Check sheet for the modelled part. Datum: model origin and axes. Units: mm. A direction names the side the tool comes from. Give positions to 0.01 mm unless a question says otherwise; leave off trailing zeros. Order: outer loops, then holes, each group sorted by start corner. A loop starts at its lowest first (then second) coordinate and runs counter-clockwise, first axis right, second up.
from build123d import *

# Parameters (mm, degrees)
F1_DEPTH  = 114.3
F2_DEPTH  = 12.7
F4_DEPTH  = 6.35
F5_W      = 6.35
F5_H      = 6.35
F6_DEPTH  = 6.35
F7_W      = 6.35
F7_H      = 6.35
F8_DEPTH  = 6.35
F9_R      = 2.5
F10_DEPTH = 6.35
F11_R     = 2.5
F12_DEPTH = 6.35
F13_W     = 6.35
F13_H     = 6.35
F14_DEPTH = 6.35


with BuildPart() as f1:
    # F0 (on Front) → F1 (new body)
    with BuildSketch(Plane.XZ):
        Polygon((45.4323484187, 0), (22.7161742094, 39.3455678842), (-22.7161742094, 39.3455678842), (-45.4323484187, 0), (-22.7161742094, -39.3455678842), (22.7161742094, -39.3455678842), align=None)
        Polygon((38.1, 0), (19.05, -32.9955678842), (-19.05, -32.9955678842), (-38.1, 0), (-19.05, 32.9955678842), (19.05, 32.9955678842), align=None, mode=Mode.SUBTRACT)
    extrude(amount=F1_DEPTH)

    # F0 (on Front) → F2 (join)
    with BuildSketch(Plane.XZ):
        Polygon((45.4323484187, 0), (22.7161742094, 39.3455678842), (-22.7161742094, 39.3455678842), (-45.4323484187, 0), (-22.7161742094, -39.3455678842), (22.7161742094, -39.3455678842), align=None)
        Polygon((38.1, 0), (19.05, -32.9955678842), (-19.05, -32.9955678842), (-38.1, 0), (-19.05, 32.9955678842), (19.05, 32.9955678842), align=None, mode=Mode.SUBTRACT)
    extrude(amount=-F2_DEPTH)

    # F3 (on Front) → F4 (join)
    with BuildSketch(Plane.XZ):
        Polygon((19.05, -32.9955678842), (38.1, 0), (19.05, 32.9955678842), (-19.05, 32.9955678842), (-38.1, 0), (-19.05, -32.9955678842), align=None)
    extrude(amount=F4_DEPTH)

    # F5 (on face) → F6 (cut)
    with BuildSketch(Plane(origin=(34.074261314, 0, 19.6727839421), x_dir=(0, 1, 0), z_dir=(0.8660254038, 0, 0.5))):
        with Locations((-111.125, 0)):
            Rectangle(F5_W, F5_H)
    extrude(amount=-F6_DEPTH, mode=Mode.SUBTRACT)

    # F7 (on face) → F8 (cut)
    with BuildSketch(Plane(origin=(-34.074261314, 0, -19.6727839421), x_dir=(0, -1, 0), z_dir=(-0.8660254038, 0, -0.5))):
        with Locations((111.125, 0)):
            Rectangle(F7_W, F7_H)
    extrude(amount=-F8_DEPTH, mode=Mode.SUBTRACT)

    # F9 (on face) → F10 (cut)
    with BuildSketch(Plane(origin=(-34.074261314, 0, -19.6727839421), x_dir=(0, -1, 0), z_dir=(-0.8660254038, 0, -0.5))):
        with Locations((38.1, 0)):
            Circle(F9_R)
    extrude(amount=-F10_DEPTH, mode=Mode.SUBTRACT)

    # F11 (on face) → F12 (cut)
    with BuildSketch(Plane(origin=(34.074261314, 0, 19.6727839421), x_dir=(0, 1, 0), z_dir=(0.8660254038, 0, 0.5))):
        with Locations((-38.1, 0)):
            Circle(F11_R)
        with Locations((-25.4, 0)):
            Circle(F11_R)
    extrude(amount=-F12_DEPTH, mode=Mode.SUBTRACT)

    # F13 (on face) → F14 (cut)
    with BuildSketch(Plane(origin=(34.074261314, 0, 19.6727839421), x_dir=(0, 1, 0), z_dir=(0.8660254038, 0, 0.5))):
        with Locations((9.525, 0)):
            Rectangle(F13_W, F13_H)
    extrude(amount=-F14_DEPTH, mode=Mode.SUBTRACT)


solid = f1.part
1) Section check C-C, the plane z = -5. Record the cut outline in (x, y), then the cut area to 3 significant figures.
Recorded:
outline: (-42.55, -114.3) - (-35.21, -114.3) - (-35.21, -6.35) - (35.21, -6.35) - (35.21, -114.3) - (42.55, -114.3) - (42.55, 12.7) - (35.21, 12.7) - (35.21, 0) - (-35.21, 0) - (-35.21, 12.7) - (-42.55, 12.7) - close
area: 2,310 mm2
2) Draft check along X on faces 4 (the face through (29.78, -111.17, 20.86)), 5 (the face through (32.951, 9.481, 15.358)), 6 (the face through (-33.915, -51.689, 19.948)). Enter one of: +X half, -X half, draft (parallel to the pull), parting line (faces both ways), or undercut.
Recorded:
face 4: +X half
face 5: undercut
face 6: -X half
3) Set-up check for faces 1 (the face through (34.23, -51.69, 19.4)), 2 (the face through (28.708, 6.261, -16.267)), 3 (the face through (-1, -6.35, 0)): record each of +Z, -Z, +X, -X, +Y, -Y from which the full face is reachable in a straight line by a thin tool's end or side.
Recorded:
face 1: +Z, +X, +Y, -Y
face 2: +Y
face 3: -Y
4) Section check A-A, the plane y = -76. Record the cut outline in (x, z).
Recorded:
outline: (-45.43, 0) - (-22.72, -39.35) - (22.72, -39.35) - (45.43, 0) - (22.72, 39.35) - (-22.72, 39.35) - close; hole (-38.1, 0) - (-19.05, -33) - (19.05, -33) - (38.1, 0) - (19.05, 33) - (-19.05, 33) - close
5) Material ranges on L1, parallel to Z at x = -8.5, y = -60; L2, parallel to Y at x = -7, z = -2.5; L3, parallel to Z at x = 20, y = -56.5, recorded low to high.
Recorded:
L1: z = -39.35 to -33, 33 to 39.35
L2: y = -6.35 to 0
L3: z = -39.35 to -31.35, 31.35 to 39.35
6) Section check B-B, the plane x = 4. Record the cut outline in (y, z).
Recorded:
outline: (-114.3, -39.35) - (12.7, -39.35) - (12.7, -33) - (0, -33) - (0, 33) - (12.7, 33) - (12.7, 39.35) - (-114.3, 39.35) - (-114.3, 33) - (-6.35, 33) - (-6.35, -33) - (-114.3, -33) - close
7) Depth check by flat-ended pin: pin 1 Ø1.5 at (y, z) = (-21.5, -1) entering from +X; pin 2 Ø2 at (x, y) = (-30, -5) entering from -Z; pin 3 Ø1.5 at (x, y) = (32.5, -39.5) entering from -Z. Enter the tip coordinate at first touch or a pass-through.
Recorded:
pin 1: stops at x = 45.29
pin 2: stops at z = -28.46
pin 3: stops at z = -23.7
